Autodesk Inventor part; units mm, degrees
ref_plane "YZ Plane" through (0, 0, 0) normal (1, 0, 0) x (0, 1, 0)
ref_plane "XZ Plane" through (0, 0, 0) normal (0, 1, 0) x (-1, 0, 0)
ref_plane "XY Plane" through (0, 0, 0) normal (0, 0, 1) x (1, 0, 0)
sketch "スケッチ1" plane through (0, 0, 0) normal (0, 0, 1) x (1, 0, 0)
  circle A0 centre (0, 0) radius 10.5 construction
  circle A1 centre (-13.5, 1) radius 1.35
  line L0 (-13.5, 28) -> (13.5, 28) construction
  line L1 (13.5, 28) -> (13.5, 1) construction
  line L2 (13.5, 1) -> (-13.5, 1) construction
  line L3 (-13.5, 1) -> (-13.5, 28) construction
  circle A2 centre (-13.5, 28) radius 1.35
  circle A3 centre (13.5, 1) radius 1.35
  circle A4 centre (13.5, 28) radius 1.35
  line L4 (-19.75, 10) -> (-19.75, 7.1)
  line L5 (-19.75, 10) -> (19.75, 10)
  line L6 (19.75, 10) -> (19.75, 7.1)
  line L7 (-19.75, -7.1) -> (-19.75, -10)
  line L8 (-19.75, -10) -> (19.75, -10)
  line L9 (19.75, -7.1) -> (19.75, -10)
  line L10 (-19.75, 5) -> (-21.75, 5)
  line L11 (-21.75, 5) -> (-21.75, -5)
  line L12 (-21.75, -5) -> (-19.75, -5)
  arc A5 (-19.75, 5) -> (-19.75, 7.1) centre (-19.75, 6.05) ccw
  arc A6 (-19.75, -7.1) -> (-19.75, -5) centre (-19.75, -6.05) ccw
  line L13 (19.75, 5) -> (21.75, 5)
  line L14 (21.75, 5) -> (21.75, -5)
  line L15 (21.75, -5) -> (19.75, -5)
  arc A7 (19.75, 7.1) -> (19.75, 5) centre (19.75, 6.05) ccw
  line L16 (0, 28) -> (0, 0) construction
  arc A8 (19.75, -5) -> (19.75, -7.1) centre (19.75, -6.05) ccw
  line L17 (-21.75, 0) -> (21.75, 0) construction
  circle A9 centre (0, 0) radius 6.05
  point P0 (0, 10)
  dimension "d8" = 21
  dimension "d10" = 27
  dimension "d12" = 1
  dimension "d13" = 2.7
  dimension "d38" = 27
  dimension "d44" = 27
  dimension "d47" = 1.05
  dimension "d48" = 39.5
  dimension "d49" = 2
  dimension "d50" = 10
  dimension "d51" = 5
  dimension "d52" = 12.1
extrude "押し出し1" add sketch "スケッチ1" along normal blind 2 contours L5 L6 A7 L13 L14 L15 A8 L9 L8 L7 A6 L12 L11 L10 A5 L4
sketch "スケッチ2" plane through (0, 0, 2) normal (0, 0, 1) x (1, 0, 0)
  circle A0 centre (0, 0) radius 6.05
  circle A1 centre (-13.5, 1) radius 1.35
  line L0 (-19.75, -10) -> (19.75, -10)
  line L1 (19.75, 10) -> (-19.75, 10)
  line L2 (-11.8485, 3) -> (-7.4162, 3)
  arc A2 (7.4162, 3) -> (-7.4162, 3) centre (0, 0) ccw
  line L3 (7.4162, 3) -> (11.8485, 3)
  line L4 (-18.4641, 12.448) -> (18.4641, 12.448)
  line L5 (-18.4641, 12.448) -> (-11.8485, 3)
  line L6 (11.8485, 3) -> (18.4641, 12.448)
  line L7 (-11.8485, -3) -> (-7.4162, -3)
  line L8 (-11.8485, -3) -> (-24.333, -20.8295)
  line L9 (-24.333, -20.8295) -> (24.333, -20.8295)
  line L10 (11.8485, -3) -> (7.4162, -3)
  line L11 (11.8485, -3) -> (24.333, -20.8295)
  arc A3 (-7.4162, -3) -> (7.4162, -3) centre (0, 0) ccw
  line L12 (-21.75, 5) -> (-21.75, -5)
  line L13 (-16.75, 10) -> (-19.75, 10) construction
  line L14 (0, 0) -> (-21.75, 0) construction
  line L15 (-19.75, -10) -> (-16.75, -10) construction
  line L16 (-19.75, -10) -> (19.75, -10) construction
  line L17 (0, 0) -> (0, 10) construction
  line L18 (19.75, 10) -> (16.75, 10) construction
  line L19 (19.75, -10) -> (16.75, -10) construction
  circle A4 centre (-13.5, 1) radius 2.5 construction
  dimension "d57" = 8
  dimension "d58" = 3
  dimension "d60" = 6
  dimension "d64" = 3
  dimension "d65" = 5
extrude "押し出し2" cut sketch "スケッチ2" against normal blind 10 contours L8 L7 A3 L10 L11 L0 | L0 L11 L9 L8 | L6 L3 A2 L2 L5 L1 | L1 L5 L4 L6
fillet "フィレット1" radius 2 12 edges at (-11.8485, 3, 1) (-7.4162, 3, 1) (7.4162, 3, 1) (11.8485, -3, 1) (7.4162, -3, 1) (-7.4162, -3, 1) (-11.8485, -3, 1) (-16.75, -10, 1) (-16.75, 10, 1) (16.75, 10, 1) (16.75, -10, 1) (11.8485, 3, 1)
sketch "スケッチ3" plane through (0, 0, 0) normal (0, 0, -1) x (-1, 0, 0)
  circle A0 centre (13.5, 1) radius 1.35
  circle A1 centre (13.5, 1) radius 1.35
  circle A2 centre (-13.5, 1) radius 1.35
  circle A3 centre (-13.5, 1) radius 1.35
  point P0 (0, 0)
extrude "押し出し3" add sketch "スケッチ3" against normal up to surface (2 mm away)
equation "\"d38\" = d10"
equation "\"d44\" = d10"
equation "\"d50\" = d11"
equation "\"d51\" = d28"
equation "\"d60\" = 2 * d58"
properties part number "足首_サブフレーム_1_2" material "アルミニウム 2014-T4"
Verification items for the finished model (mm, model axes). A direction names the side the tool comes from. Give positions to 0.01 mm unless a question says otherwise; leave off trailing zeros. Order: outer loops, then holes, each group sorted by start corner. A loop starts at its lowest first (then second) coordinate and runs counter-clockwise, first axis right, second up. Notation, with made-up numbers: (45.25, 41.5) -> (53.25, 41.5) arc R30 cw to (53.25, 69.5) -> close; hole circle Ø9 at (19.25, 3). An arc over 180 degrees is marked (long way). Use a Markdown table: item, result.
1) Material ranges on probe 1 along X at (y, z) = (6.5, 0.1); probe 2 along X at (y, z) = (-3.5, 1.7); probe 3 along X at (y, z) = (5.5, 1), recorded low to high.
Results:
| item | result |
|---|---|
| probe 1 | -18.8 to -14.3, -4.66 to 4.66, 14.3 to 18.8 |
| probe 2 | -21.75 to -12.13, -7.34 to -4.93, 4.93 to 7.34, 12.13 to 21.75 |
| probe 3 | -18.86 to -13.6, -5.81 to -2.52, 2.52 to 5.81, 13.6 to 18.86 |
2) Section check B-B, the plane y = 0. Record the boundary of the cut face in (x, z).
Results:
| item | result |
|---|---|
| outline | (-21.75, 0) -> (-6.05, 0) -> (-6.05, 2) -> (-21.75, 2) -> close; (6.05, 0) -> (21.75, 0) -> (21.75, 2) -> (6.05, 2) -> close |
3) Section check C-C, the plane x = 12. Record the boundary of the cut face in (y, z), then the cut area to 3 significant figures.
Results:
| item | result |
|---|---|
| outline | (-3.39, 0) -> (3.39, 0) -> (3.39, 2) -> (-3.39, 2) -> close |
| area | 13.6 mm² |
4) Section check A-A, the plane x = 0. Record the boundary of the cut face in (y, z), then the cut area to 3 significant figures.
Results:
| item | result |
|---|---|
| outline | (-8, 0) -> (-6.05, 0) -> (-6.05, 2) -> (-8, 2) -> close; (6.05, 0) -> (8, 0) -> (8, 2) -> (6.05, 2) -> close |
| area | 7.80 mm² |
5) Depth check by flat-ended pin: pin 1 Ø0.6 at (y, z) = (8.5, 1.5) entering from -X; pin 2 Ø1 at (x, z) = (9.5, 1.5) entering from -Y; pin 3 Ø0.6 at (x, z) = (21, 0.5) entering from -Y. Enter the tip coordinate at first touch or a pass-through.
Results:
| item | result |
|---|---|
| pin 1 | x = -19.75 |
| pin 2 | y = -3 |
| pin 3 | y = -5 |
6) Tool access check on faces 1 (the cylindrical face through (-7.673, -3.261, 0.986)), 2 (the flat face through (-21, 5, 1)), 3 (the flat face through (-21, -5, 1)). Record the directions out of +Z, -Z, +X, -X, +Y, -Y that give a thin tool (end or side, any length) a straight path to the whole face; none if there is none.
Results:
| item | result |
|---|---|
| face 1 | +Z, -Z, -Y |
| face 2 | +Z, -Z, -X, +Y |
| face 3 | +Z, -Z, -X, -Y |
7) Mould release check, pull along Y, two halves, no side actions. Record for faces 4 (the cylindrical face through (16.86, -9.77, 1.01)), 5 (the flat face through (21, 5, 1)), 6 (the cylindrical face through (-18.7, 6.1, 1)): pulls with the +Y half, pulls with the -Y half, needs draft (parallel to the pull), parting line crosses it, or undercut.
Results:
| item | result |
|---|---|
| face 4 | pulls with the -Y half |
| face 5 | pulls with the +Y half |
| face 6 | undercut |
